CAD build for the part. Positions are in the model's coordinates, mm. A direction names the side the tool comes from. Coordinates: 2 decimals unless noted, no trailing zeros. Loops run counter-clockwise (first coordinate to the right, second up) from the corner with the lowest first, then second, coordinate; pieces in that order, holes last. Notation, with made-up numbers: (68.25, -2.75) -> (92.25, -2.75) arc R13 ccw to (92.25, 19.25) -> close; hole circle Ø8 at (82, -16.75). An arc over 180 degrees is marked (long way). Answer as a JSON object with one key per item and string values. Group by question number.
Autodesk Inventor part; units mm, degrees
ref_plane "YZ Plane" through (0, 0, 0) normal (1, 0, 0) x (0, 1, 0)
ref_plane "XZ Plane" through (0, 0, 0) normal (0, 1, 0) x (-1, 0, 0)
ref_plane "XY Plane" through (0, 0, 0) normal (0, 0, 1) x (1, 0, 0)
sketch "Sketch1" plane through (0, 0, 0) normal (0, 1, 0) x (-1, 0, 0)
  arc A0 (-2.75, 2.1651) -> (2.75, 2.1651) centre (0, 0) ccw
  line L0 (-1.9, 14.1) -> (-2.75, 2.1651)
  line L1 (1.8987, 14.0987) -> (2.75, 2.1651)
  arc A1 (1.8987, 14.0987) -> (-1.9, 14.1) centre (-0.0007, 14.05) ccw
  circle A2 centre (0, 0) radius 0.5
  line L2 (0, 0) -> (0, -10) construction
  line L3 (0, 30) -> (0, 0) construction
  arc A3 (-7.6535, 3.6978) -> (7.6533, 3.6982) centre (0, 0) ccw
  line L4 (7.6533, 3.6982) -> (6.8916, 14.3762)
  arc A4 (6.8916, 14.3762) -> (-6.8928, 14.3783) centre (-0.0007, 14.05) ccw
  line L5 (-6.8928, 14.3783) -> (-7.6535, 3.6978)
  line L6 (10, 0) -> (-10, 0)
  line L7 (-10, 0) -> (-10, 30)
  line L8 (-10, 30) -> (10, 30)
  line L9 (10, 30) -> (10, 0)
  point P0 (-8.5, 0)
  point P1 (8.5, 0)
  dimension "d0" = 1
  dimension "d9" = 1.9
  dimension "d11" = 3.5
  dimension "d34" = 10
  dimension "d42" = 5
  dimension "d43" = 20
  dimension "d44" = 30
extrude "Extrusion6" add sketch "Sketch1" along normal blind 8 contours A0 L6 A3 L5 A4 L4 L1 A1 L0 | A0 L6 A3 | L6 L7 L8 L9 A3 L4 A4 L5
sketch "Sketch7" plane through (0, 0, 0) normal (0, -1, 0) x (1, 0, 0)
  arc A0 (-8.5, 0) -> (8.5, 0) centre (0, 0) ccw
  line L0 (10, 30) -> (10, 0)
  line L1 (-10, 0) -> (-10, 30)
  line L2 (-10, 0) -> (-10, 30)
  line L3 (-10, 0) -> (-7.225, -4.4777)
  line L4 (10, 0) -> (7.225, -4.4777)
  line L5 (8.5, 0) -> (10, 0)
  line L6 (-8.5, 0) -> (-10, 0)
  line L7 (-8.5, 0) -> (-10, 0)
extrude "Extrusion7" add sketch "Sketch7" against normal blind 8
fillet "Fillet1" radius 5 2 edges at (10, 4, 0) (-10, 4, 0)
sketch "Sketch8" plane through (0, 0, 0) normal (0, -1, 0) x (1, 0, 0)
  arc A0 (-10, 1.4237) -> (-9.25, -1.2102) centre (-5, 1.4237) ccw
  line L0 (-9.25, -1.2102) -> (-7.225, -4.4777)
  arc A1 (-7.225, -4.4777) -> (7.225, -4.4777) centre (0, 0) ccw
  line L1 (7.225, -4.4777) -> (9.25, -1.2102)
  arc A2 (9.25, -1.2102) -> (10, 1.4237) centre (5, 1.4237) ccw
  line L2 (10, 30) -> (10, 1.4237)
  line L3 (-10, 30) -> (10, 30)
  line L4 (-10, 1.4237) -> (-10, 30)
  arc A3 (-2.75, 2.1651) -> (2.75, 2.1651) centre (0, 0) ccw
  line L5 (-1.8987, 14.0987) -> (-2.75, 2.1651)
  arc A4 (1.9, 14.1) -> (-1.8987, 14.0987) centre (0.0007, 14.05) ccw
  line L6 (2.75, 2.1651) -> (1.9, 14.1)
  circle A5 centre (0, 20) radius 10
  line L7 (10, 30) -> (10, 1.4237)
  line L8 (-10, 30) -> (10, 30)
  point P0 (-10, 20)
  point P1 (0, 30)
  point P2 (10, 20)
  dimension "d50" = 20
extrude "Extrusion8" cut sketch "Sketch8" against normal through all contours L4 L3 A5 | L3 L2 A5
sketch "Sketch9" plane through (0, 8, 0) normal (0, 1, 0) x (1, 0, 0)
  arc A0 (-10, -20) -> (10, -20) centre (0, -20) ccw
  line L0 (-10, -1.4237) -> (-10, -20)
  arc A1 (-9.25, 1.2102) -> (-10, -1.4237) centre (-5, -1.4237) ccw
  line L1 (-7.225, 4.4777) -> (-9.25, 1.2102)
  arc A2 (7.225, 4.4777) -> (-7.225, 4.4777) centre (0, 0) ccw
  line L2 (9.25, 1.2102) -> (7.225, 4.4777)
  arc A3 (10, -1.4237) -> (9.25, 1.2102) centre (5, -1.4237) ccw
  line L3 (10, -20) -> (10, -1.4237)
extrude "Extrusion9" add sketch "Sketch9" against normal blind 5
properties part number "Servo_Shaft_select_V1"
Item 1: Band-saw the part on B-B, the plane y = 5.25. List the corners of the cut face in (x, z) (3 decimals).
Item 2: Drill centre lines: L1, parallel to X at y = 2.5, z = -2; L2, parallel to X at y = 1.5, z = 0; L3, parallel to Z at x = -1.5, y = 2. Where is each one in solid material? Low to high.
Item 3: Band-saw the part on D-D, the plane x = -4.25. List the corners of the cut face in (y, z).
Item 4: Flat gauge pins, fed straight in: P1, Ø3, axis at x = 5.5, z = 18, coming from the -Y side; P2, Ø1.5, axis at x = 7.5, y = 3, coming from the +Z side; P3, Ø1.5, axis at y = 5, z = -2.5, coming from the +X side. Where does each tip first touch, or does it go through?
Item 5: Band-saw the part on C-C, the plane y = 1. List the corners of the cut face in (x, z) (3 decimals).
Item 6: Pull direction X, two halves, no side cores. Call faces 3 (the flat face through (-10, 4, 11)), 4 (the flat face through (10, 4, 11)), 5 (the flat face through (0, 3, 6)): +X half, -X half, draft (parallel to the pull), parting line (faces both ways), or undercut.
Item 7: Band-saw the part on A-A, the plane x = 0. List the corners of the cut face in (y, z), and give its area (3 significant figures).
Item 8: 3-axis set-ups, long thin cutter, end or side, ignore diameter. For faces 1 (the flat face through (-8.25, 3.94, -2.82)), 2 (the flat face through (2.32, 1.48, 8.22)): which of +Z, -Z, +X, -X, +Y, -Y reach the whole face in a straight line?
Reply:
{
 "1": {"outline": "(-10, 1.424) arc R5 ccw to (-9.25, -1.21) -> (-7.225, -4.478) arc R8.5 ccw to (7.225, -4.478) -> (9.25, -1.21) arc R5 ccw to (10, 1.424) -> (10, 20) arc R10 ccw to (-10, 20) -> close"},
 "2": {"L1": "-8.76 to -2.87, 2.87 to 8.76", "L2": "-9.79 to -3.5, 3.5 to 9.79", "L3": "-8.37 to -3.16, 15.22 to 29.89"},
 "3": {"outline": "(0, -7.36) -> (8, -7.36) -> (8, 29.05) -> (0, 29.05) -> close"},
 "4": {"P1": "y = 0", "P2": "z = 27.38", "P3": "x = 8.92"},
 "5": {"outline": "(-10, 1.424) arc R5 ccw to (-9.25, -1.21) -> (-7.225, -4.478) arc R8.5 ccw to (7.225, -4.478) -> (9.25, -1.21) arc R5 ccw to (10, 1.424) -> (10, 20) arc R10 ccw to (-10, 20) -> close; hole (-2.75, 2.165) arc R3.5 ccw (long way) to (2.75, 2.165) -> (1.9, 14.1) arc R1.9 ccw to (-1.899, 14.099) -> close"},
 "6": {"face 3": "-X half", "face 4": "+X half", "face 5": "undercut"},
 "7": {"outline": "(0, -8.5) -> (8, -8.5) -> (8, 30) -> (0, 30) -> (0, 15.95) -> (3, 15.95) -> (3, -3.5) -> (0, -3.5) -> close", "area": "250 mm²"},
 "8": {"face 1": "-Z, -X, +Y, -Y", "face 2": "-Y"}
}
